Autodesk Fusion 360 part; units mm, degrees
sketch "Esboço1" plane through (0, 0, 0) normal (0, 0, 1) x (1, 0, 0)
  line L0 (0, 0) -> (120, 0)
  line L1 (120, 0) -> (120, 35)
  line L2 (120, 35) -> (0, 35)
  line L3 (0, 35) -> (0, 0)
  dimension "d1" = 120
  dimension "d2" = 35
extrude "Extrusão1" add sketch "Esboço1" along normal blind 4
sketch "Esboço2" plane through (0, 0, 4) normal (0, 0, 1) x (-1, 0, 0)
  line L0 (0, -35) -> (0, 0)
  line L1 (0, 0) -> (-120, 0)
  line L2 (-120, 0) -> (-120, -35)
  line L3 (-120, -35) -> (0, -35)
  line L4 (-10, -30) -> (-110, -30)
  line L5 (-110, -30) -> (-110, -5)
  line L6 (-110, -5) -> (-10, -5)
  line L7 (-10, -5) -> (-10, -30)
  point P0 (-5, -30)
  point P1 (-5, -5)
  point P2 (-115, -5)
  point P3 (-115, -30)
extrude "Extrusão2" add sketch "Esboço2" along normal blind 5 contours L4 L5 L6 L7
sketch "Esboço3" plane through (0, 0, 9) normal (0, 0, 1) x (-1, 0, 0)
  line L0 (-10, -5) -> (-110, -5)
  line L1 (-110, -5) -> (-110, -30)
  line L2 (-110, -30) -> (-10, -30)
  line L3 (-10, -30) -> (-10, -5)
sketch "Esboço4" plane through (110, 0, 0) normal (1, 0, 0) x (0, 1, 0)
  line L0 (5, 4) -> (30, 4)
  line L1 (30, 4) -> (30, 9)
  line L2 (30, 9) -> (5, 9)
  line L3 (5, 9) -> (5, 4)
  line L4 (5, 9) -> (5, 8)
  line L5 (30, 9) -> (30, 8)
  line L6 (5, 8) -> (30, 8)
  line L7 (6, 8) -> (6, 5)
  line L8 (6, 5) -> (29, 5)
  line L9 (29, 5) -> (29, 8)
extrude "Extrusão3" cut sketch "Esboço4" against normal blind 95 contours L6 L7 L8 L9
sketch "Esboço5" plane through (0, 0, 9) normal (0, 0, 1) x (1, 0, 0)
  line L0 (110, 30) -> (110, 23)
  line L1 (110, 5) -> (110, 12)
  line L2 (110, 23) -> (35, 23)
  line L3 (110, 12) -> (35, 12)
  line L4 (35, 12) -> (35, 23)
  line L5 (110, 23) -> (110, 12)
  dimension "d9" = 7
  dimension "d10" = 7
extrude "Extrusão4" cut sketch "Esboço5" against normal blind 5
sketch "Esboço6" plane through (0, 0, 4) normal (0, 0, 1) x (1, 0, 0)
extrude "Extrusão5" add 1 faces at (35, 15.6667, 4.3333) along direction (1, 0, 0) blind 75
sketch "Esboço7" plane through (110, 0, 0) normal (1, 0, 0) x (0, 1, 0)
  line L0 (5, 4) -> (30, 4)
  line L1 (30, 4) -> (30, 9)
  line L2 (30, 9) -> (23, 9)
  line L3 (23, 9) -> (23, 8)
  line L4 (23, 8) -> (29, 8)
  line L5 (29, 8) -> (29, 5)
  line L6 (29, 5) -> (6, 5)
  line L7 (6, 5) -> (6, 8)
  line L8 (6, 8) -> (12, 8)
  line L9 (12, 8) -> (12, 9)
  line L10 (12, 9) -> (5, 9)
  line L11 (5, 9) -> (5, 4)
  line L12 (6, 8) -> (29, 8)
  line L13 (29, 8) -> (29, 8.3)
  line L14 (29, 8.3) -> (6, 8.3)
  line L15 (6, 8.3) -> (6, 8)
  dimension "d15" = 0.3
extrude "Extrusão6" add sketch "Esboço7" against normal blind 75 contours L3 L9 L12 L14
sketch "Esboço8" plane through (0, 0, 4) normal (0, 0, 1) x (1, 0, 0)
  circle A0 centre (5, 30) radius 2
  circle A1 centre (5, 5) radius 2
  circle A2 centre (115, 30) radius 2
  circle A3 centre (115, 5) radius 2
  dimension "d18" = 4
  dimension "d19" = 4
  dimension "d20" = 4
  dimension "d21" = 4
extrude "Extrusão7" cut sketch "Esboço8" against normal blind 20
sketch "Esboço9" plane through (10, 0, 0) normal (-1, 0, 0) x (0, -1, 0)
  line L0 (-30, 4) -> (-5, 4)
  line L1 (-5, 4) -> (-5, 9)
  line L2 (-5, 9) -> (-30, 9)
  line L3 (-30, 9) -> (-30, 4)
  line L4 (-30, 9) -> (-31.5, 9)
  line L5 (-31.5, 9) -> (-31.5, 4)
  line L6 (-31.5, 4) -> (-30, 4)
  line L7 (-30, 4) -> (-30, 9)
  line L8 (-5, 9) -> (-3.5, 9)
  line L9 (-3.5, 9) -> (-3.5, 4)
  line L10 (-3.5, 4) -> (-5, 4)
  line L11 (-5, 4) -> (-5, 9)
  dimension "d24" = 1.5
  dimension "d25" = 1.5
  dimension "d26" = 5
extrude "Extrusão8" add sketch "Esboço9" against normal blind 100 contours L3 L4 L5 L6 L7 | L1 L8 L9 L10 L11
extrude "Extrusão9" add 1 faces at (18.3333, 19.3333, 9) along direction (0, 0, 1) blind 1.2
chamfer "Chanfro1" distance 1 angle 50 1 edges at (110, 17.5, 5) measured on face at (110, 4.3333, 7.4)
equation "d24 = ( 0.3 * 5 ) * 1 mm"
equation "d25 = ( 0.3 * 5 ) * 1 mm"
equation "d29 = ( 0.3 * 4 ) * 1 mm"
The listing builds one solid part. Answer for the finished solid, in the listing's coordinates (mm). A direction names the side the tool comes from. Coordinates: 2 decimals unless noted, no trailing zeros. Write each loop counter-clockwise with the first axis right and the second up, starting at its lowest first coordinate (ties: lowest second). Pieces come first, ordered by that corner, then holes. Notation, with made-up numbers: (83, -24.5) - (117, -24.5) arc R15 cw to (117, -12.5) - close; hole circle Ø9 at (-9, 43.25). An arc over 180 degrees is marked (long way). Return JSON: item names as keys, results as strings. Group by question number.
Q1. Which of the six approach directions +Z, -Z, +X, -X, +Y, -Y give full straight-line access (tool end or side, diameter ignored) to faces 4 (the flat face through (73, 23, 9)), 5 (the flat face through (59, 31.5, 7)), 6 (the flat face through (15, 17, 7)), 7 (the flat face through (59, 3.5, 7)), 8 (the flat face through (10, 18, 7))?
Q2. For a pull along X with two mould halves and no side action, classify faces 1 (the cylindrical face through (5, 28, 2)), 2 (the flat face through (110, 23.9, 8.4)), 3 (the flat face through (63, 17, 8)) as +X half, -X half, draft (parallel to the pull), parting line (faces both ways), or undercut.
Q3. Flat-ended cylindrical pins translate along their axes: pin 1 Ø2.5 at (y, z) = (14.5, 6) entering from +X; pin 2 Ø4 at (x, z) = (106, 5.5) entering from -Y; pin 3 Ø1.9 at (x, z) = (37.5, 7.5) entering from +Y; pin 4 Ø1.9 at (x, z) = (45, 8) entering from -Y. Find the tip coordinate at first contact, or state that the pin passes through.
Q4. The part is cut by section C-C on x = 115. Write down the section's boundary in (y, z).
Q5. Find the intervals of material crossed by line 1 along Y through (x, z) = (5, 1.55); line 2 along Z through (x, y) = (75, 26); line 3 along Z through (x, y) = (42.5, 15), in increasing order. Write a range as [from, to].
Q6. The part is cut by section D-D on z = 6.25. Write down the section's boundary in (x, y), and give its area (3 significant figures).
Q7. The part is cut by section A-A on x = 47.5. Write down the section's boundary in (y, z).
Evaluation:
{
 "1": {"face 4": "+Z, +X", "face 5": "+Z, +X, -X, +Y", "face 6": "+X", "face 7": "+Z, +X, -X, -Y", "face 8": "+Z, -X, +Y, -Y"},
 "2": {"face 1": "undercut", "face 2": "+X half", "face 3": "draft"},
 "3": {"pin 1": "stops at x = 109.11", "pin 2": "stops at y = 0", "pin 3": "stops at y = 31.5", "pin 4": "stops at y = 3.5"},
 "4": {"outline": "(0, 0) - (3, 0) - (3, 4) - (0, 4) - close; (7, 0) - (28, 0) - (28, 4) - (7, 4) - close; (32, 0) - (35, 0) - (35, 4) - (32, 4) - close"},
 "5": {"line 1": "y = [0, 3], [7, 28], [32, 35]", "line 2": "z = [0, 5], [8, 10.2]", "line 3": "z = [0, 5], [8, 8.3]"},
 "6": {"outline": "(10, 3.5) - (110, 3.5) - (110, 6) - (15, 6) - (15, 29) - (110, 29) - (110, 31.5) - (10, 31.5) - close", "area": "615 mm2"},
 "7": {"outline": "(0, 0) - (35, 0) - (35, 4) - (31.5, 4) - (31.5, 10.2) - (23, 10.2) - (23, 8.3) - (12, 8.3) - (12, 10.2) - (3.5, 10.2) - (3.5, 4) - (0, 4) - close; hole (6, 5) - (29, 5) - (29, 8) - (6, 8) - close"}
}
